```python
from build123d import *

# Parameters (mm, degrees)
SKETCH1_R           = 3
BOSS_EXTRUDE1_DEPTH = 12
SKETCH2_R           = 4.5
BOSS_EXTRUDE2_DEPTH = 3
CUT_EXTRUDE3_START  = -3
CUT_EXTRUDE3_DEPTH  = 3
SKETCH4_OUTSIDE_W   = 49.116
SKETCH4_OUTSIDE_H   = 47.938
SKETCH4_OUTSIDE_R   = 3.895
CUT_EXTRUDE4_DEPTH  = 17.141517221
CUT_EXTRUDE4_DRAFT  = -45


with BuildPart() as part:
    # Sketch1 → Boss-Extrude1 (new body)
    with BuildSketch(Plane(origin=(0, 0, 0), x_dir=(1, 0, 0), z_dir=(0, 1, 0))):
        with Locations(Location((0, 0, 0), (0, 0, 270))):
            Circle(SKETCH1_R)
    extrude(amount=BOSS_EXTRUDE1_DEPTH)

    # Sketch2 → Boss-Extrude2 (add)
    with BuildSketch(Plane(origin=(0, 12, 0), x_dir=(1, 0, 0), z_dir=(0, 1, 0))):
        with Locations(Location((0, 0, 0), (0, 0, 270))):
            Circle(SKETCH2_R)
    extrude(amount=BOSS_EXTRUDE2_DEPTH)

    # Sketch3 → Cut-Extrude3 (cut)
    with BuildSketch(Plane(origin=(0, 15, 0), x_dir=(1, 0, 0), z_dir=(0, 1, 0)).offset(CUT_EXTRUDE3_START)):
        with BuildLine():
            ThreePointArc((-4.499907692, 0.028823035), (-3.911445893, -2.224992365), (-2.274915326, -3.882622858))
            Line((-2.274915326, -3.882622858), (-4.499907692, 0.028823035))
        make_face()
        with BuildLine():
            ThreePointArc((-2.224992365, 3.911445893), (-3.882622858, 2.274915326), (-4.499907692, 0.028823035))
            Line((-4.499907692, 0.028823035), (-2.224992365, 3.911445893))
        make_face()
        with BuildLine():
            Line((-2.224992365, 3.911445893), (2.274915326, 3.882622858))
            ThreePointArc((2.274915326, 3.882622858), (0.028823035, 4.499907692), (-2.224992365, 3.911445893))
        make_face()
        with BuildLine():
            Line((2.274915326, 3.882622858), (4.499907692, -0.028823035))
            ThreePointArc((4.499907692, -0.028823035), (4.499976923, -0.014411591), (4.5, 0))
            ThreePointArc((4.5, 0), (3.904300127, 2.237507657), (2.274915326, 3.882622858))
        make_face()
        with BuildLine():
            Line((4.499907692, -0.028823035), (2.224992365, -3.911445893))
            ThreePointArc((2.224992365, -3.911445893), (3.882622858, -2.274915326), (4.499907692, -0.028823035))
        make_face()
        with BuildLine():
            ThreePointArc((-2.274915326, -3.882622858), (-0.028823035, -4.499907692), (2.224992365, -3.911445893))
            Line((2.224992365, -3.911445893), (-2.274915326, -3.882622858))
        make_face()
    extrude(amount=CUT_EXTRUDE3_DEPTH, mode=Mode.SUBTRACT)


with BuildPart() as cut_extrude4_tool:
    # Sketch4 outside → Cut-Extrude4 (with draft: the straight prism first)
    with BuildSketch(Plane(origin=(0, 15, 0), x_dir=(1, 0, 0), z_dir=(0, 1, 0))):
        Rectangle(SKETCH4_OUTSIDE_W, SKETCH4_OUTSIDE_H)
        Circle(SKETCH4_OUTSIDE_R, mode=Mode.SUBTRACT)
    extrude(amount=-CUT_EXTRUDE4_DEPTH)
    # Cut-Extrude4: the draft: its side faces are tilted about the plane it starts from
    cut_extrude4_sides = [cut_extrude4_tool.faces().sort_by_distance(p)[0] for p in [
        (0, 6.429241389, 23.969),
        (24.558, 6.429241389, 0),
        (0, 6.429241389, -23.969),
        (-24.558, 6.429241389, 0),
        (-3.895, 6.429241389, 0),
    ]]
    draft(cut_extrude4_sides, Plane(origin=(0, 15, 0), x_dir=(1, 0, 0), z_dir=(0, 1, 0)), CUT_EXTRUDE4_DRAFT)


with BuildPart() as part_1:
    add(part.part)

    # Cut-Extrude4: cut by cut_extrude4_tool
    add(cut_extrude4_tool.part, mode=Mode.SUBTRACT)


solid = part_1.part
```
Model file for the job. Use its own axes, mm. A direction names the side the tool comes from. Give positions to 0.01 mm unless a question says otherwise; leave off trailing zeros. Order: outer loops, then holes, each group sorted by start corner. A loop starts at its lowest first (then second) coordinate and runs counter-clockwise, first axis right, second up.
1) 3-axis set-ups, long thin cutter, end or side, ignore diameter. For faces 1 (the cylindrical face through (0.9, 5.92, 2.86)), 2 (the flat face through (-3.372, 13.478, 1.954)): which of +Z, -Z, +X, -X, +Y, -Y reach the whole face in a straight line?
2) Wall check: probe 1 along Y at (x, z) = (-2.75, 2.25); probe 2 along Z at (x, y) = (-2.75, 13.25); probe 3 along Z at (x, y) = (-4, 14.25). Give the ranges that are in metal, low to high.
3) Saw through at B-B, the plane y = 5.75. Write the cut outline in (x, z).
4) Pin check, flat tips, straight feed: pin 1 (1 mm diameter, centred on y = 10, z = 1.5, fed in from -X); pin 2 (3 mm diameter, centred on y = 3.5, z = 1.5, fed in from -X). Stop position of each tip, or through.
Computed:
1. face 1: -Y
1. face 2: +Z, -X, +Y, -Y
2. probe 1: y = 12 to 15
2. probe 2: z = -3.02 to 3.05
2. probe 3: z = -0.88 to 0.85
3. outline: circle Ø6 at (0, 0)
4. pin 1: stops at x = -2.83
4. pin 2: stops at x = -3
